Work out the finished part from the listing and answer in its coordinate system (mm). A direction names the side the tool comes from. Round coordinates to 2 decimals unless told otherwise and drop trailing zeros. Write each loop counter-clockwise with the first axis right and the second up, starting at its lowest first coordinate (ties: lowest second). Pieces come first, ordered by that corner, then holes. Notation, with made-up numbers: (-19, 56.25) - (17, 56.25) arc R25 cw to (17, 75.25) - close; hole circle Ø4 at (37.5, 49.5). An arc over 180 degrees is marked (long way). Write item = value, one per line. Start each with the question number.
Solid Edge part; units mm, degrees
sketch "Sketch1" plane through (0, 0, 0) normal (0, 0, -1) x (-1, 0, 0)
  line L0 (95.3397, -103.6479) -> (51.2285, -77.4874)
  arc A0 (50.1607, -73.407) -> (51.2285, -77.4874) centre (52.7588, -74.907) ccw
  line L1 (50.1607, -73.407) -> (87.8058, -8.2038)
  arc A1 (87.8058, -8.2038) -> (93.1692, -6.7667) centre (91.2061, -10.1669) cw
  line L2 (93.1692, -6.7667) -> (141.6312, -34.7462)
  arc A2 (152.148, -28.6744) -> (141.6312, -34.7462) centre (145.1368, -28.6744) cw
  line L3 (152.148, -28.6744) -> (152.148, 41.3592)
  line L4 (152.148, 41.3592) -> (152.148, 56.9741)
  arc A3 (152.148, 56.9741) -> (149.6578, 67.5392) centre (128.4914, 56.9741) ccw
  line L5 (149.6578, 67.5392) -> (143.3974, 80.0815)
  line L6 (143.3974, 80.0815) -> (139.7875, 87.3136)
  arc A4 (132.4553, 96.1265) -> (139.7875, 87.3136) centre (117.3845, 76.1313) cw
  line L7 (132.4553, 96.1265) -> (115.6366, 108.8032)
  line L8 (115.6366, 108.8032) -> (47.4442, 148.174)
  arc A5 (47.4442, 148.174) -> (38.9522, 143.2712) centre (44.6135, 143.2712) ccw
  line L9 (38.9522, 143.2712) -> (38.9522, 82.3207)
  arc A6 (35.9522, 79.3207) -> (38.9522, 82.3207) centre (35.9522, 82.3207) ccw
  line L10 (35.9522, 79.3207) -> (0, 79.3207)
  line L11 (-35.9522, 79.3207) -> (0, 79.3207)
  arc A7 (-38.9522, 82.3207) -> (-35.9522, 79.3207) centre (-35.9522, 82.3207) ccw
  line L12 (-38.9522, 143.2712) -> (-38.9522, 82.3207)
  arc A8 (-47.4442, 148.174) -> (-38.9522, 143.2712) centre (-44.6135, 143.2712) cw
  line L13 (-115.6366, 108.8032) -> (-47.4442, 148.174)
  line L14 (-133.5716, 95.2852) -> (-115.6366, 108.8032)
  arc A9 (-139.1633, 88.5642) -> (-133.5716, 95.2852) centre (-122.0781, 80.0363) cw
  line L15 (-143.3974, 80.0815) -> (-139.1633, 88.5642)
  line L16 (-146.6042, 73.6569) -> (-143.3974, 80.0815)
  arc A10 (-152.148, 50.1368) -> (-146.6042, 73.6569) centre (-99.4833, 50.1368) cw
  line L17 (-152.148, 41.3592) -> (-152.148, 50.1368)
  line L18 (-152.148, -28.6744) -> (-152.148, 41.3592)
  arc A11 (-152.148, -28.6744) -> (-140.9818, -35.1212) centre (-144.7038, -28.6744) ccw
  line L19 (-92.869, -7.3433) -> (-140.9818, -35.1212)
  arc A12 (-92.869, -7.3433) -> (-87.4547, -8.794) centre (-90.8872, -10.7758) cw
  line L20 (-49.853, -73.922) -> (-87.4547, -8.794)
  arc A13 (-49.853, -73.922) -> (-50.9511, -78.0201) centre (-52.4511, -75.422) cw
  line L21 (-95.3397, -103.6479) -> (-50.9511, -78.0201)
  line L22 (-104.033, -108.8682) -> (-95.3397, -103.6479)
  arc A14 (-104.3735, -113.774) -> (-104.033, -108.8682) centre (-102.4886, -111.4401) cw
  line L23 (-98.2167, -118.7465) -> (-104.3735, -113.774)
  line L24 (-98.2167, -118.7465) -> (-70.6434, -125.0511)
  line L25 (-70.6434, -125.0511) -> (0, -125.0511)
  line L26 (70.6434, -125.0511) -> (0, -125.0511)
  line L27 (98.2167, -118.7465) -> (70.6434, -125.0511)
  line L28 (98.2167, -118.7465) -> (104.3735, -113.774)
  arc A15 (104.033, -108.8682) -> (104.3735, -113.774) centre (102.4886, -111.4401) cw
  line L29 (104.033, -108.8682) -> (95.3397, -103.6479)
  line L30 (39.0877, 12.7232) -> (39.0877, -61.8289)
  line L31 (39.0877, -61.8289) -> (24.621, -75.4447)
  line L32 (24.621, -75.4447) -> (0, -75.4447)
  line L33 (-24.621, -75.4447) -> (0, -75.4447)
  line L34 (-39.0877, -61.8289) -> (-24.621, -75.4447)
  line L35 (-39.0877, 12.7232) -> (-39.0877, -61.8289)
  line L36 (-42.2177, 12.7232) -> (-39.0877, 12.7232)
  line L37 (-42.2177, 56.9983) -> (-42.2177, 12.7232)
  line L38 (0, 56.9983) -> (-42.2177, 56.9983)
  line L39 (0, 56.9983) -> (42.2177, 56.9983)
  line L40 (42.2177, 56.9983) -> (42.2177, 12.7232)
  line L41 (42.2177, 12.7232) -> (39.0877, 12.7232)
extrude "Protrusion1" add sketch "Sketch1" against normal blind 1.6
hole "Hole_1" at (-61.8402, -103.4888, 1.6) direction (0, 0, -1) diameter 3.5 end up to next
hole "Hole1" at (61.7723, -103.4888, 1.6) direction (0, 0, -1) diameter 3.5 end up to next
hole "Hole2" at (-80.0108, 10.0358, 1.6) direction (0, 0, -1) diameter 3.5 end up to next
hole "Hole3" at (79.9982, 10.0358, 1.6) direction (0, 0, -1) diameter 3.5 end up to next
hole "Hole4" at (43.2229, 105.2486, 1.6) direction (0, 0, -1) diameter 3.5 end up to next
hole "Hole5" at (-43.264, 105.3035, 1.6) direction (0, 0, -1) diameter 3.5 end up to next
hole "Hole6" at (139.1633, 76.8692, 1.6) direction (0, 0, -1) diameter 3.5 end up to next
hole "Hole7" at (-139.7875, 76.8692, 1.6) direction (0, 0, -1) diameter 3.5 end up to next
1. Find section D-D on z = 1.3. Give the number of separate pieces and of enclosed holes in the cut face, plus the area to 3 significant figures.
2. Find section B-B on x = -14.5. Give the vertices of the cut face in (y, z), plus the area to 3 significant figures.
3. Find section A-A on y = 37. Give the vertices of the cut face in (x, z).
4. Which of the six approach directions +Z, -Z, +X, -X, +Y, -Y give full straight-line access (tool end or side, diameter ignored) to faces 1 (the face through (73.456, -91.013, 0.789)), 2 (the face through (-117.06, -20.56, 0.79)), 3 (the face through (-73.59, -90.75, 0.79)), 4 (the face through (2, 75, 1.6))?
5. Each of these flat-tipped pins is pushed along its axis until it touches: pin 1 (0.5 mm diameter, centred on y = 112, z = 0.5, fed in from +X); pin 2 (0.8 mm diameter, centred on x = -41, z = 0.5, fed in from +Y); pin 3 (0.8 mm diameter, centred on y = 126, z = 1, fed in from -X). Where does it stop, or does it pass through?
6. Consider line 1 (X direction, y = -18.5, z = 1.1); line 2 (X direction, y = -14, z = 1.35); line 3 (Y direction, x = 14.5, z = 0.75). Determine where each line is inside the solid, lowest interval first.
7. Find section C-C on y = -21.5. Give the vertices of the cut face in (x, z), plus the area to 3 significant figures.
8. For a pull along X with two mould halves and no side action, classify faces 5 (the face through (-32, -68.5, 0.8)), 6 (the face through (2, 75, 0)), 7 (the face through (82.02, 128.21, 0.79)) as released by +X, released by -X, zero draft, split by the parting line, or undercut.
Answer key:
q1.separate_pieces = 1
q1.enclosed_holes = 9
q1.area = 44,000 mm²
q2.outline = (-125.05, 0) - (-75.44, 0) - (-75.44, 1.6) - (-125.05, 1.6) - close; (57, 0) - (79.32, 0) - (79.32, 1.6) - (57, 1.6) - close
q2.area = 115 mm²
q3.outline = (-152.15, 0) - (-42.22, 0) - (-42.22, 1.6) - (-152.15, 1.6) - close; (42.22, 0) - (152.15, 0) - (152.15, 1.6) - (42.22, 1.6) - close
q4.face_1 = +Z, -Z, +X
q4.face_2 = +Z, -Z
q4.face_3 = +Z, -Z, -X
q4.face_4 = +Z, +X, -X, +Y, -Y
q5.pin_1 = 110.53
q5.pin_2 = 147.93
q5.pin_3 = -86.54
q6.line_1 = -152.15 to -113.49, -81.86 to -39.09, 39.09 to 81.85, 112.19 to 152.15
q6.line_2 = -152.15 to -105.7, -84.46 to -39.09, 39.09 to 84.45, 104.4 to 152.15
q6.line_3 = -125.05 to -75.44, 57 to 79.32
q7.outline = (-152.15, 0) - (-118.69, 0) - (-118.69, 1.6) - (-152.15, 1.6) - close; (-80.13, 0) - (-39.09, 0) - (-39.09, 1.6) - (-80.13, 1.6) - close; (39.09, 0) - (80.12, 0) - (80.12, 1.6) - (39.09, 1.6) - close; (117.39, 0) - (152.15, 0) - (152.15, 1.6) - (117.39, 1.6) - close
q7.area = 240 mm²
q8.face_5 = undercut
q8.face_6 = zero draft
q8.face_7 = released by +X
